from build123d import *

# Parameters (mm, degrees)
SKETCH1_W           = 254
SKETCH1_H           = 381
BOSS_EXTRUDE1_DEPTH = 203.2
SHELL1_T            = -3.175
CUT_EXTRUDE1_REACH  = 378.957
SKETCH2_R           = 14.25
CUT_EXTRUDE2_REACH  = 378.957
SKETCH3_R           = 14.25
SKETCH4_W           = 152.4
SKETCH4_H           = 12.7
BOSS_EXTRUDE2_DEPTH = 127
CUT_EXTRUDE3_REACH  = 420.33
SKETCH5_R           = 38.1
FILLET1_R           = 25.4
FILLET2_R           = 25.4
CUT_EXTRUDE4_REACH  = 308.12
SKETCH6_R           = 6.35
SKETCH6_R_2         = 12.5


with BuildPart() as part:
    # Sketch1 → Boss-Extrude1 (new body)
    with BuildSketch(Plane(origin=(0, 0, 0), x_dir=(1, 0, 0), z_dir=(0, 1, 0))):
        Rectangle(SKETCH1_W, SKETCH1_H)
    extrude(amount=BOSS_EXTRUDE1_DEPTH)

    # Shell1
    shell1_openings = [part.faces().sort_by_distance(p)[0] for p in [
        (0, 203.2, 0),
    ]]
    offset(amount=SHELL1_T, openings=shell1_openings, kind=Kind.INTERSECTION)

    # Sketch2 → Cut-Extrude1 (cut, up to next)
    with BuildSketch(Plane(origin=(127, 0, 0), x_dir=(0, 0, -1), z_dir=(1, 0, 0)), mode=Mode.PRIVATE) as cut_extrude1_sk1:
        with Locations((-114.3, 142.875)):
            Circle(SKETCH2_R)
    cut_extrude1_tool1 = extrude(cut_extrude1_sk1.sketch, amount=-CUT_EXTRUDE1_REACH, mode=Mode.PRIVATE) & part.part
    # Sketch2 → Cut-Extrude1 (cut, up to next)
    with BuildSketch(Plane(origin=(127, 0, 0), x_dir=(0, 0, -1), z_dir=(1, 0, 0)), mode=Mode.PRIVATE) as cut_extrude1_sk2:
        with Locations((-114.3, 60.325)):
            Circle(SKETCH2_R)
    cut_extrude1_tool2 = extrude(cut_extrude1_sk2.sketch, amount=-CUT_EXTRUDE1_REACH, mode=Mode.PRIVATE) & part.part
    add(cut_extrude1_tool1.solids().sort_by_distance((127, 142.875, 114.3))[0], mode=Mode.SUBTRACT)
    add(cut_extrude1_tool2.solids().sort_by_distance((127, 60.325, 114.3))[0], mode=Mode.SUBTRACT)

    # Sketch3 → Cut-Extrude2 (cut, up to next)
    with BuildSketch(Plane.ZY.offset(127), mode=Mode.PRIVATE) as cut_extrude2_sk1:
        with Locations((-127, 142.875)):
            Circle(SKETCH3_R)
    cut_extrude2_tool1 = extrude(cut_extrude2_sk1.sketch, amount=-CUT_EXTRUDE2_REACH, mode=Mode.PRIVATE) & part.part
    # Sketch3 → Cut-Extrude2 (cut, up to next)
    with BuildSketch(Plane.ZY.offset(127), mode=Mode.PRIVATE) as cut_extrude2_sk2:
        with Locations((-127, 60.325)):
            Circle(SKETCH3_R)
    cut_extrude2_tool2 = extrude(cut_extrude2_sk2.sketch, amount=-CUT_EXTRUDE2_REACH, mode=Mode.PRIVATE) & part.part
    add(cut_extrude2_tool1.solids().sort_by_distance((-127, 142.875, -127))[0], mode=Mode.SUBTRACT)
    add(cut_extrude2_tool2.solids().sort_by_distance((-127, 60.325, -127))[0], mode=Mode.SUBTRACT)

    # Sketch4 → Boss-Extrude2 (add)
    with BuildSketch(Plane.XZ):
        with Locations((0, -146.05)):
            Rectangle(SKETCH4_W, SKETCH4_H)
    extrude(amount=BOSS_EXTRUDE2_DEPTH)

    # Sketch5 → Cut-Extrude3 (cut, up to next)
    with BuildSketch(Plane(origin=(0, 0, -152.4), x_dir=(-1, 0, 0), z_dir=(0, 0, -1)), mode=Mode.PRIVATE) as cut_extrude3_sk1:
        with Locations((0, -76.2)):
            Circle(SKETCH5_R)
    cut_extrude3_tool1 = extrude(cut_extrude3_sk1.sketch, amount=-CUT_EXTRUDE3_REACH, mode=Mode.PRIVATE) & part.part
    add(cut_extrude3_tool1.solids().sort_by_distance((0, -76.2, -152.4))[0], mode=Mode.SUBTRACT)

    # Fillet1
    fillet1_edges = [part.edges().sort_by_distance(p)[0] for p in [
        (-76.2, -127, -146.05),
        (76.2, -127, -146.05),
    ]]
    fillet(fillet1_edges, radius=FILLET1_R)

    # Fillet2
    fillet2_edges = [part.edges().sort_by_distance(p)[0] for p in [
        (0, 0, -139.7),
    ]]
    fillet(fillet2_edges, radius=FILLET2_R)

    # Sketch6 → Cut-Extrude4 (cut, up to next)
    with BuildSketch(Plane.XZ, mode=Mode.PRIVATE) as cut_extrude4_sk1:
        with Locations(Location((63.5, 165.1, 0), (0, 0, 270))):
            Circle(SKETCH6_R)
    cut_extrude4_tool1 = extrude(cut_extrude4_sk1.sketch, amount=-CUT_EXTRUDE4_REACH, mode=Mode.PRIVATE) & part.part
    # Sketch6 → Cut-Extrude4 (cut, up to next)
    with BuildSketch(Plane.XZ, mode=Mode.PRIVATE) as cut_extrude4_sk2:
        with Locations(Location((-88.9, -63.5, 0), (0, 0, 270))):
            Circle(SKETCH6_R_2)
    cut_extrude4_tool2 = extrude(cut_extrude4_sk2.sketch, amount=-CUT_EXTRUDE4_REACH, mode=Mode.PRIVATE) & part.part
    # Sketch6 → Cut-Extrude4 (cut, up to next)
    with BuildSketch(Plane.XZ, mode=Mode.PRIVATE) as cut_extrude4_sk3:
        with Locations(Location((101.6, -160.02, 0), (0, 0, 270))):
            Circle(SKETCH6_R_2)
    cut_extrude4_tool3 = extrude(cut_extrude4_sk3.sketch, amount=-CUT_EXTRUDE4_REACH, mode=Mode.PRIVATE) & part.part
    add(cut_extrude4_tool1.solids().sort_by_distance((63.5, 0, 165.1))[0], mode=Mode.SUBTRACT)
    add(cut_extrude4_tool2.solids().sort_by_distance((-88.9, 0, -63.5))[0], mode=Mode.SUBTRACT)
    add(cut_extrude4_tool3.solids().sort_by_distance((101.6, 0, -160.02))[0], mode=Mode.SUBTRACT)


solid = part.part
Can you work these out from the model? Positions are in its coordinate system, mm. A direction names the side the tool comes from. Round coordinates to 2 decimals unless told otherwise and drop trailing zeros. Loops run counter-clockwise (first coordinate to the right, second up) from the corner with the lowest first, then second, coordinate; pieces in that order, holes last. Notation, with made-up numbers: (5, 57) - (57, 57) arc R15 ccw to (57, 68) - close; hole circle Ø8 at (-20.75, 56). An arc over 180 degrees is marked (long way). Answer in a Markdown table with one row per item. Add a question column.
Q1. I want a section at B-B on x = 101.6. List the corners of the cut face in (y, z) for me (3 decimals).
Q2. Which directions (+Z, -Z, +X, -X, +Y, -Y) give clear straight access to the entire face, cutting with the end or side of a thin tool? Please do faces 4 (the flat face through (-76.2, -50, -146)), 5 (the flat face through (127, 100, 3)), 6 (the flat face through (76.2, -50, -146)), 7 (the flat face through (-123.825, 102, 3)), 8 (the cylindrical face through (4.96, -38.424, -146.139)).
Q3. We'd pull the mould along Y, two halves only. Please class faces 1 (the flat face through (-2, 100, -190.5)), 2 (the flat face through (-1, -127, -146)), 3 (the cylindrical face through (-125.435, 54.867, -113.837)): pulls with the +Y half, pulls with the -Y half, needs draft (parallel to the pull), parting line crosses it, or undercut.
Q4. For pin 1 Ø4 at (x, z) = (40.5, 97) entering from -Y; pin 2 Ø20 at (x, z) = (101.6, -160.02) entering from -Y; pin 3 Ø11.5 at (y, z) = (-52.5, -139) entering from +X; pin 4 Ø19 at (y, z) = (-62, -140.5) entering from -X, each with a flat end and sliding along its axis, tell me the tip position at first contact or that it passes through.
Q5. I want a section at D-D on z = -127. List the corners of the cut face in (x, y) for me (3 decimals), and give its area (3 significant figures).
Q6. I want a section at C-C on z = 165.1. List the corners of the cut face in (x, y) for me (3 decimals).
Q7. I want a section at A-A on y = -76.2. List the corners of the cut face in (x, z) for me, and give its area (3 significant figures).
Q8. I need wall thicknesses on L1, parallel to Y at x = 124.8, z = 114.3 (3 decimals); L2, parallel to Z at x = -72, y = 92 (3 decimals); L3, parallel to X at y = 88.5, z = 26.5 (3 decimals). Which ranges of each line are inside material? Lowest first, please.
A:
| question | item | result |
|---|---|---|
| 1 | outline | (0, -190.5) - (203.2, -190.5) - (203.2, -187.325) - (3.175, -187.325) - (3.175, -172.52) - (0, -172.52) - close; (0, -147.52) - (3.175, -147.52) - (3.175, 187.325) - (203.2, 187.325) - (203.2, 190.5) - (0, 190.5) - close |
| 2 | face 4 | +Z, -Z, -X, -Y |
| 2 | face 5 | +Z, -Z, +X, +Y, -Y |
| 2 | face 6 | +Z, -Z, +X, -Y |
| 2 | face 7 | +Y |
| 2 | face 8 | +Z, -Z |
| 3 | face 1 | needs draft |
| 3 | face 2 | pulls with the -Y half |
| 3 | face 3 | undercut |
| 4 | pin 1 | y = 0 |
| 4 | pin 2 | through |
| 4 | pin 3 | x = 76.2 |
| 4 | pin 4 | x = -76.2 |
| 5 | outline | (-127, 0) - (-76.2, 0) - (-76.2, -3.403) - (76.2, -3.403) - (76.2, 0) - (127, 0) - (127, 203.2) - (123.825, 203.2) - (123.825, 3.175) - (-123.825, 3.175) - (-123.825, 46.075) - (-127, 46.075) - close; (-127, 74.575) - (-123.825, 74.575) - (-123.825, 128.625) - (-127, 128.625) - close; (-127, 157.125) - (-123.825, 157.125) - (-123.825, 203.2) - (-127, 203.2) - close |
| 5 | area | 2,410 mm^2 |
| 6 | outline | (-127, 0) - (57.15, 0) - (57.15, 3.175) - (-123.825, 3.175) - (-123.825, 203.2) - (-127, 203.2) - close; (69.85, 0) - (127, 0) - (127, 203.2) - (123.825, 203.2) - (123.825, 3.175) - (69.85, 3.175) - close |
| 7 | outline | (-76.2, -152.4) - (-38.1, -152.4) - (-38.1, -139.7) - (-76.2, -139.7) - close; (38.1, -152.4) - (76.2, -152.4) - (76.2, -139.7) - (38.1, -139.7) - close |
| 7 | area | 968 mm^2 |
| 8 | L1 | 0 to 46.075, 74.575 to 128.625, 157.125 to 203.2 |
| 8 | L2 | -190.5 to -187.325, 187.325 to 190.5 |
| 8 | L3 | -127 to -123.825, 123.825 to 127 |
